Geometry check sheet. Reference: the model listing, model coordinates, mm. Face numbers are marked on the shaded views. A direction names the side the tool comes from. Give positions to 0.01 mm unless a question says otherwise; leave off trailing zeros. Loops run counter-clockwise (first coordinate to the right, second up) from the corner with the lowest first, then second, coordinate; pieces in that order, holes last. Notation, with made-up numbers: (89, 60.5) -> (94, 60.5) arc R14 cw to (94, 65.5) -> close; hole circle Ø6 at (78, 16). An arc over 180 degrees is marked (long way). One line per question, with ' | ' between items.
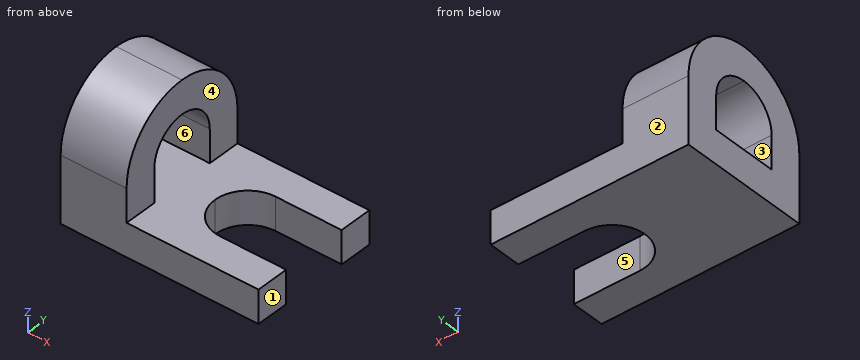
from build123d import *

# Parameters (mm, degrees)
F1_DEPTH = 50.8
F2_W     = 50.8
F2_H     = 50.8
F3_DEPTH = 204.4911384583
F4_W     = 76.2
F4_H     = 50.8
F5_DEPTH = 61.3817144185
F6_R     = 50.79999
F7_R     = 25.39999
F8_R     = 25.39999


# Not quite as in the source:
# - a fillet or chamfer is up to 0.001 mm smaller than in the source, because OpenCascade refuses the exact size


with BuildPart() as f1:
    # F0 (on Front) → F1 (new body, symmetric)
    with BuildSketch(Plane.XZ):
        Polygon((-25.4, -25.4), (-25.4, 50.8), (-76.2, 50.8), (-76.2, -50.8), (76.2, -50.8), (76.2, -25.4), align=None)
    extrude(amount=F1_DEPTH, both=True)

    # F2 (on face) → F3 (cut)
    with BuildSketch(Plane.YZ.offset(-25.4)):
        Rectangle(F2_W, F2_H)
    extrude(amount=-F3_DEPTH, mode=Mode.SUBTRACT)

    # F4 (on face) → F5 (cut)
    with BuildSketch(Plane.XY.offset(-25.4)):
        with Locations((38.1, 0)):
            Rectangle(F4_W, F4_H)
    extrude(amount=-F5_DEPTH, mode=Mode.SUBTRACT)

    # F6 (radius 50.8 in the source; OpenCascade refuses exactly that, so slightly less here)
    f6_edges = [f1.edges().sort_by_distance(p)[0] for p in [
        (-50.8, -50.8, 50.8),
        (-50.8, 50.8, 50.8),
    ]]
    fillet(f6_edges, radius=F6_R)

    # F7 (radius 25.4 in the source; OpenCascade refuses exactly that, so slightly less here)
    f7_edges = [f1.edges().sort_by_distance(p)[0] for p in [
        (-50.8, -25.4, 25.4),
        (-50.8, 25.4, 25.4),
    ]]
    fillet(f7_edges, radius=F7_R)

    # F8 (radius 25.4 in the source; OpenCascade refuses exactly that, so slightly less here)
    f8_edges = [f1.edges().sort_by_distance(p)[0] for p in [
        (0, -25.4, -38.1),
        (0, 25.4, -38.1),
    ]]
    fillet(f8_edges, radius=F8_R)


solid = f1.part
Item 1: Release check for a two-part mould opening along Y. For the marked faces 1, 2 and 3 record: pulls with the +Y half, pulls with the -Y half, needs draft (parallel to the pull), parting line crosses it, or undercut.
Result:
face 1: needs draft | face 2: pulls with the +Y half | face 3: undercut
Item 2: Set-up check for the marked faces 4, 5 and 6: record each of +Z, -Z, +X, -X, +Y, -Y from which the full face is reachable in a straight line by a thin tool's end or side.
Result:
face 4: +Z, +X, +Y, -Y | face 5: +Z, -Z, +X | face 6: +X, -X
Item 3: Depth check by flat-ended pin: pin 1 Ø12 at (y, z) = (-18, 19.5) entering from +X; pin 2 Ø3 at (x, z) = (43.5, -23.5) entering from -Y. Enter the tip coordinate at first touch or a pass-through.
Result:
pin 1: x = -25.4 | pin 2: through
Item 4: Sectioned sample at A-A (x = 63). Record the cut outline in (y, z), plus the area to 3 significant figures.
Result:
outline: (-50.8, -50.8) -> (-25.4, -50.8) -> (-25.4, -25.4) -> (-50.8, -25.4) -> close; (25.4, -50.8) -> (50.8, -50.8) -> (50.8, -25.4) -> (25.4, -25.4) -> close | area: 1,290 mm2
Item 5: Sectioned sample at B-B (z = -17.5). Record the cut outline in (x, y), plus the area to 3 significant figures.
Result:
outline: (-76.2, -50.8) -> (-25.4, -50.8) -> (-25.4, -25.4) -> (-76.2, -25.4) -> close; (-76.2, 25.4) -> (-25.4, 25.4) -> (-25.4, 50.8) -> (-76.2, 50.8) -> close | area: 2,580 mm2
Item 6: Scan lines: probe 1 along X at (y, z) = (42, -17.5); probe 2 along Y at (x, z) = (51.5, -36); probe 3 along Y at (x, z) = (-32.5, 5). Record each from-to range of solid material in increasing order.
Result:
probe 1: -76.2 to -25.4 | probe 2: -50.8 to -25.4, 25.4 to 50.8 | probe 3: -50.55 to -24.9, 24.9 to 50.55
